Solid Edge part; units mm, degrees
sketch "Sketch1" plane through (0, 0, 0) normal (0, -1, 0) x (1, 0, 0)
  line L0 (-46.526, 0) -> (-5.526, 0)
  arc A0 (-5.526, 4) -> (-5.526, 0) centre (-5.526, 2) cw
  line L1 (-5.526, 4) -> (-46.526, 4)
  arc A1 (-46.526, 0) -> (-46.526, 4) centre (-46.526, 2) cw
  circle A2 centre (-46.526, 2) radius 0.95
  circle A3 centre (-5.526, 2) radius 0.95
extrude "Protrusion1" add sketch "Sketch1" along normal mid plane 2
properties material "Stainless Steel, 420"
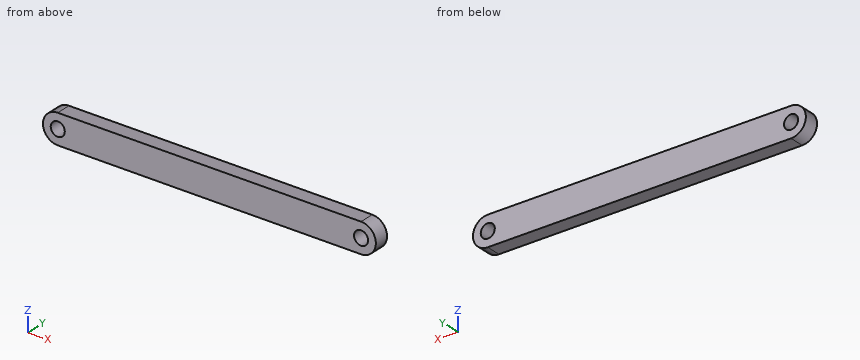
Could you check a few things on this model? Use its own coordinates, in mm. Round coordinates to 2 decimals unless told otherwise and drop trailing zeros. Order: outer loops, then holes, each group sorted by start corner. A loop starts at its lowest first (then second) coordinate and runs counter-clockwise, first axis right, second up.
(1) Please list where these lines run through material, in increasing order: line 1 along X through (y, z) = (0.35, 2.3); line 2 along X through (y, z) = (-0.7, 1); line 3 along X through (y, z) = (0.65, 3.4).
Response values:
line 1: x = -48.5 to -47.43, -45.62 to -6.43, -4.62 to -3.55
line 2: x = -48.26 to -3.79
line 3: x = -47.95 to -4.1
(2) Imagine slicing it at B-B (y = 0.4). Write out the boundary of the cut face in (x, z).
Response values:
outline: (-46.53, 0) - (-5.53, 0) arc R2 ccw to (-5.53, 4) - (-46.53, 4) arc R2 ccw to start; hole circle Ø1.9 at (-46.53, 2); hole circle Ø1.9 at (-5.53, 2)
(3) I'm going to push a flat-ended pin straight in: pin 1 (2 mm diameter, centred on x = -5.526, z = 2, fed in from +Y). Where does the tip first touch, or does it pass through?
Response values:
pin 1: stops at y = 1
(4) Imagine slicing it at A-A (z = 2). Write out the boundary of the cut face in (x, y).
Response values:
outline: (-48.53, -1) - (-47.48, -1) - (-47.48, 1) - (-48.53, 1) - close; (-45.58, -1) - (-6.48, -1) - (-6.48, 1) - (-45.58, 1) - close; (-4.58, -1) - (-3.53, -1) - (-3.53, 1) - (-4.58, 1) - close
